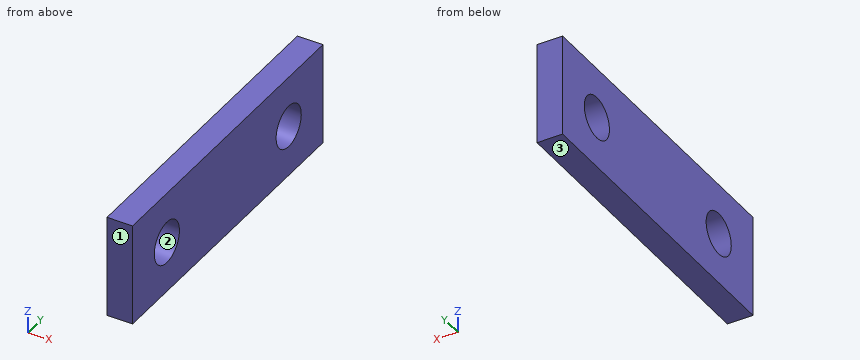
from build123d import *

# Parameters (mm, degrees)
SKETCH1_W           = 125
SKETCH1_H           = 40
SKETCH1_R           = 8.25
BOSS_EXTRUDE1_DEPTH = 5


with BuildPart() as part:
    # Sketch1 → Boss-Extrude1 (new, symmetric)
    with BuildSketch(Plane.YZ):
        Rectangle(SKETCH1_W, SKETCH1_H)
        with Locations(Location((-40, 0, 0), (0, 0, 270))):
            Circle(SKETCH1_R, mode=Mode.SUBTRACT)
        with Locations(Location((40, 0, 0), (0, 0, 270))):
            Circle(SKETCH1_R, mode=Mode.SUBTRACT)
    extrude(amount=BOSS_EXTRUDE1_DEPTH, both=True)


solid = part.part
Design review of the part built by this model. Coordinates are the model's own, in mm. Face numbers are marked on the shaded views. Coordinates: 2 decimals unless noted, no trailing zeros. Loops run counter-clockwise (first coordinate to the right, second up) from the corner with the lowest first, then second, coordinate; pieces in that order, holes last. Notation, with made-up numbers: M -10,63 L 25,63 A14 ccw 25,75 Z; hole C 19.25,46.25 d5. An arc over 180 degrees is marked long. Answer as CSV lines item,"result".
Item 1: The part is to be moulded in two halves that separate along Z. For the marked faces 1, 2 and 3, say which applies: pulls with the +Z half, pulls with the -Z half, needs draft (parallel to the pull), parting line crosses it, or undercut.
Answer list:
face 1,"needs draft"
face 2,"undercut"
face 3,"pulls with the -Z half"
Item 2: Add section C-C on x = -2.5. State the section outline as (y, z) points.
Answer list:
outline,"M -62.5,-20 L 62.5,-20 L 62.5,20 L -62.5,20 Z; hole C -40,0 d16.5; hole C 40,0 d16.5"
Item 3: For probe 1 along Y at (x, z) = (1.75, 0); probe 2 along Y at (x, z) = (1.5, -1.5); probe 3 along Z at (x, y) = (4, 39.5), list the stretches that pass through material, from the lowest coordinate up.
Answer list:
probe 1,"-62.5 to -48.25, -31.75 to 31.75, 48.25 to 62.5"
probe 2,"-62.5 to -48.11, -31.89 to 31.89, 48.11 to 62.5"
probe 3,"-20 to -8.23, 8.23 to 20"
Item 4: Add section A-A on z = 0. State the section outline as (x, y) points.
Answer list:
outline,"M -5,-62.5 L 5,-62.5 L 5,-48.25 L -5,-48.25 Z; M -5,-31.75 L 5,-31.75 L 5,31.75 L -5,31.75 Z; M -5,48.25 L 5,48.25 L 5,62.5 L -5,62.5 Z"
Item 5: Add section D-D on y = 43. State the section outline as (x, z) points.
Answer list:
outline,"M -5,-20 L 5,-20 L 5,-7.69 L -5,-7.69 Z; M -5,7.69 L 5,7.69 L 5,20 L -5,20 Z"
Item 6: For P1, Ø10, axis at y = -40, z = 0, coming from the +X side, flat-tipped, find the tip position at first contact; note if it passes through.
Answer list:
P1,"through"
Item 7: Add section B-B on y = -40. State the section outline as (x, z) points, plus the area to 3 significant figures.
Answer list:
outline,"M -5,-20 L 5,-20 L 5,-8.25 L -5,-8.25 Z; M -5,8.25 L 5,8.25 L 5,20 L -5,20 Z"
area,"235 mm²"
